Work out the finished part from the listing and answer in its coordinate system (mm). Round coordinates to 2 decimals unless told otherwise and drop trailing zeros. Order: outer loops, then holes, each group sorted by start corner. A loop starts at its lowest first (then second) coordinate and runs counter-clockwise, first axis right, second up.
from build123d import *

# Parameters (mm, degrees)
F1_DEPTH = 18.708162
F2_R     = 5.08


with BuildPart() as f1:
    # F0 (on Front) → F1 (new body)
    with BuildSketch(Plane.XZ):
        Polygon((38.234155, 52.624799), (-38.234155, 52.624799), (-61.864162, -20.100885), (0, -65.047829), (61.864162, -20.100885), align=None)
    extrude(amount=F1_DEPTH)

    # F2
    f2_edges = [f1.edges().sort_by_distance(p)[0] for p in [
        (50.049158, -18.708162, 16.261957),
        (50.049158, 0, 16.261957),
        (30.932081, -18.708162, -42.574357),
        (30.932081, 0, -42.574357),
        (-30.932081, 0, -42.574357),
        (-30.932081, -18.708162, -42.574357),
        (0, 0, 52.624799),
        (-50.049158, 0, 16.261957),
        (0, -18.708162, 52.624799),
        (-50.049158, -18.708162, 16.261957),
        (-38.234155, -9.354081, 52.624799),
        (-61.864162, -9.354081, -20.100885),
    ]]
    fillet(f2_edges, radius=F2_R)


solid = f1.part
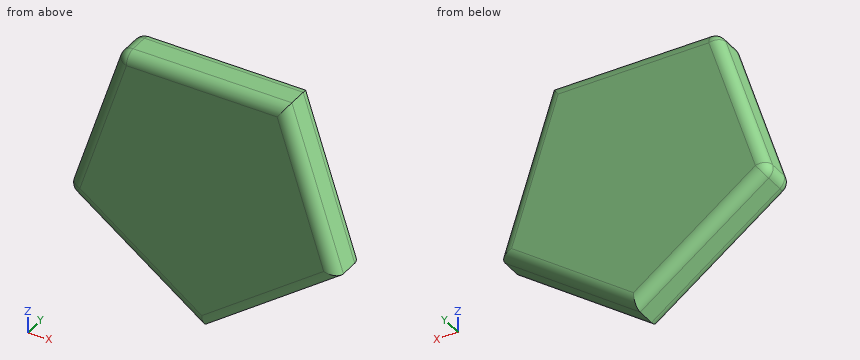
Item 1: Find section B-B (y = -2). Write down the section's boundary in (x, z).
Item 2: Find section A-A (y = -16.25). Write down the section's boundary in (x, z).
Item 3: Find the intervals of material crossed by line 1 along Z through (x, y) = (-8.5, -6.5); line 2 along X through (y, z) = (-2.75, 11); line 3 along X through (y, z) = (-1.5, 30), in increasing order.
Item 4: Given pin 1 (5 mm diameter, centred on y = -5.5, z = 21.5, fed in from +X); pin 2 (1 mm diameter, centred on x = 8.5, y = -5.5, fed in from -Z); pin 3 (1 mm diameter, centred on x = 7.5, y = -4, fed in from +Z), each flat-ended and moving along its own axis, determine where each tip first touches the part or whether it passes through.
Model answer:
1. outline: (-59.73, -16.91) arc R4.04 ccw to (-58.27, -21.43) - (0, -63.76) - (60.64, -19.7) - (37.48, 51.58) - (-34.54, 51.58) arc R4.04 ccw to (-38.39, 48.79) - close
2. outline: (-60.03, -16.82) arc R4.35 ccw to (-58.45, -21.68) - (0, -64.15) - (61.01, -19.82) - (37.7, 51.9) - (-34.54, 51.9) arc R4.35 ccw to (-38.68, 48.89) - close
3. line 1: z = -58.87 to 52.62
3. line 2: x = -51.16 to 51.16
3. line 3: x = -44.03 to 44.03
4. pin 1: stops at x = 49.16
4. pin 2: stops at z = -59.24
4. pin 3: stops at z = 52.59
